Geometry: final body of the model. Coordinates: model frame, mm. Face numbers are marked on the shaded views. Give positions to 0.01 mm unless a question says otherwise; leave off trailing zeros. Loops run counter-clockwise (first coordinate to the right, second up) from the corner with the lowest first, then second, coordinate; pieces in that order, holes last. Notation, with made-up numbers: (67.25, 8.5) -> (95.25, 8.5) arc R24 ccw to (95.25, 24.5) -> close; hole circle Ø1 at (31.25, 38). An arc over 180 degrees is marked (long way). One line per question, with ' | ' between items. Start each with the question number.
Item 1: Section B-B on z = 4.25. Return loops of the section in (x, y).
Item 2: Material intervals for line 1 along X through (y, z) = (2.7, 0); line 2 along X through (y, z) = (2.25, 0), sorted ascending. Write a range as [from, to].
Item 3: Section C-C on y = -4. Return loops of the section in (x, z), then the cut area to 3 significant figures.
Item 4: Pin query (flat end, axial travel): P1, Ø2, axis at x = 13.5, y = 2, coming from the +Z side; P2, Ø1.5, axis at x = 9.5, y = -2, coming from the +Z side; P3, Ø6, axis at x = -3, z = -2.5, coming from the -Y side; P4, Ø6, axis at x = 8.5, z = -5, coming from the -Y side. Return the tip coordinate at first contact, or that it passes through.
Item 5: Section D-D on x = 4.5. Return loops of the section in (y, z), then the cut area to 3 significant figures.
Item 6: Mould query, pull axis X, two halves, no side actions, for the marked faces 1, 2 and 3. Classes: released by +X, released by -X, zero draft, split by the parting line, or undercut.
Item 7: Section A-A on x = 0. Return loops of the section in (y, z), then the cut area to 3 significant figures.
Autodesk Inventor part; units mm, degrees
ref_plane "YZ Plane" through (0, 0, 0) normal (1, 0, 0) x (0, 1, 0)
ref_plane "XZ Plane" through (0, 0, 0) normal (0, 1, 0) x (-1, 0, 0)
ref_plane "XY Plane" through (0, 0, 0) normal (0, 0, 1) x (1, 0, 0)
sketch "Sketch2" plane through (0, 0, 0) normal (0, 1, 0) x (-1, 0, 0)
  circle A0 centre (0, 0) radius 6.269
  circle A1 centre (0, 0) radius 7.5
  dimension "d0" = 12.538
  dimension "d1" = 15
extrude "Extrusion1" add sketch "Sketch2" along normal blind 5
sketch "Sketch4" plane through (0, 5, 0) normal (0, 1, 0) x (1, 0, 0)
  circle A0 centre (0, 0) radius 7.5
  circle A1 centre (0, 0) radius 6.269
  circle A2 centre (0, 0) radius 7.5
  line L0 (7.5, 0) -> (22.5, 0)
  circle A3 centre (22.5, 0) radius 2.5
  line L1 (22.97, -2.457) -> (1.6667, -7.3125)
  line L2 (22.97, 2.457) -> (1.6667, 7.3125)
  line L3 (22.97, -2.457) -> (23.0556, -2.4375)
  line L4 (22.97, 2.457) -> (23.0556, 2.4375)
  point P0 (22.5114, 2.4471)
  point P1 (1.6667, 7.3125)
  point P2 (1.6667, -7.3125)
  point P3 (22.5114, -2.4471)
  dimension "d11" = 15
  dimension "d12" = 5
extrude "Extrusion3" add sketch "Sketch4" against normal blind 2.5 contours L0 A3 L1 A0 | A0 L2 A3 L0 | A3
sketch "Sketch5" plane through (0, 0, 0) normal (0, -1, 0) x (1, 0, 0)
  circle A0 centre (0, 0) radius 7.5
  circle A1 centre (0, 0) radius 6.269
  line L0 (0, 7.5) -> (0, -7.5)
  circle A2 centre (0, 0) radius 7.5
  point P0 (0, -6.269)
  point P1 (0, -7.5)
  point P2 (0, 6.269)
revolve "Revolution2" add sketch "Sketch5" angle 180 about axis through (0, 0, 7.5) along (0, 0, -1) picked at (6.9746, -1.0213) contours A0 L0 A1
properties part number "powderScoop_3DPrint"
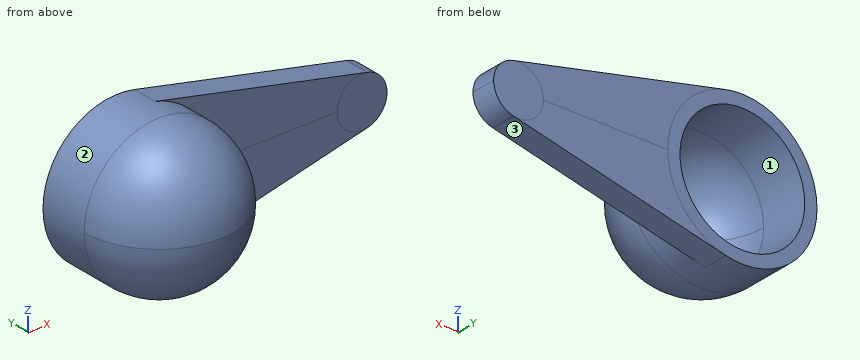
Result sheet:
1) outline: (-6.18, 0) arc R6.18 ccw to (6.18, 0) -> (6.18, 2.5) -> (15.1, 2.5) -> (15.1, 5) -> (4.61, 5) -> (4.61, 0) arc R4.61 cw to (-4.61, 0) -> (-4.61, 5) -> (-6.18, 5) -> close
2) line 1: x = [-7.5, -6.27], [6.27, 25] | line 2: x = [-7.5, -6.27], [6.27, 7.5]
3) outline: circle Ø12.69 at (0, 0); hole circle Ø9.65 at (0, 0) | area: 53.2 mm²
4) P1: stops at z = 4.81 | P2: passes through | P3: stops at y = -7.45 | P4: stops at y = -3.03
5) outline: (0, -6) -> (2.5, -6) -> (2.5, -6.67) -> (5, -6.67) -> (5, -4.36) -> (0, -4.36) arc R4.36 cw to (0, 4.36) -> (5, 4.36) -> (5, 6.67) -> (2.5, 6.67) -> (2.5, 6) -> (0, 6) arc R6 ccw to start | area: 46.3 mm²
6) face 1: undercut | face 2: split by the parting line | face 3: released by +X
7) outline: (0, -7.5) -> (5, -7.5) -> (5, -6.27) -> (0, -6.27) arc R6.27 cw to (0, 6.27) -> (5, 6.27) -> (5, 7.5) -> (0, 7.5) arc R7.5 ccw to start | area: 38.9 mm²
